Geometry check sheet. Reference: the model listing, model coordinates, mm. Face numbers are marked on the shaded views. A direction names the side the tool comes from. Coordinates: 2 decimals unless noted, no trailing zeros. Loops run counter-clockwise (first coordinate to the right, second up) from the corner with the lowest first, then second, coordinate; pieces in that order, holes last.
from build123d import *

# Parameters (mm, degrees)
F0_R        = 1.85
F0_R_2      = 15
F0_W        = 10
F0_H        = 10
F1_DEPTH    = 5
F2_DEPTH    = 22
F3_R        = 4.99999
F4_T1_DEPTH = 22
F5_R        = 1.5
F6_DEPTH    = 25


# Not quite as in the source:
# - a fillet or chamfer that OpenCascade refuses, or shapes differently, is made with other operations: its cross-section is extruded or revolved along the edge and cut away or added
# - a fillet or chamfer is up to 0.001 mm smaller than in the source, because OpenCascade refuses the exact size
# - a feature names something its author has since deleted; it is built from what else it names


with BuildPart() as f1:
    # F0 (on Top) → F1 (new body)
    with BuildSketch(Plane.XY):
        with BuildLine():
            Line((0, 15), (0, 0))
            Line((0, 0), (15, 0))
            Line((15, 0), (15, 3))
            ThreePointArc((15, 3), (8.6554793841, 7.8795661534), (5, 15))
            Line((5, 15), (0, 15))
        make_face()
        with Locations((6, 6)):
            Circle(F0_R, mode=Mode.SUBTRACT)
        with BuildLine():
            Line((15, 3), (15, 0))
            Line((15, 0), (35, 0))
            Line((35, 0), (35, 3))
            ThreePointArc((35, 3), (41.3445206159, 7.8795661534), (45, 15))
            Line((45, 15), (50, 15))
            Line((50, 15), (50, 35))
            Line((50, 35), (40, 35))
            Line((40, 35), (40, 45))
            Line((40, 45), (50, 45))
            Line((50, 45), (50, 100))
            Line((50, 100), (40, 100))
            Line((40, 100), (40, 104))
            Line((40, 104), (10, 104))
            Line((10, 104), (10, 100))
            Line((10, 100), (0, 100))
            Line((0, 100), (0, 45))
            Line((0, 45), (10, 45))
            Line((10, 45), (10, 35))
            Line((10, 35), (0, 35))
            Line((0, 35), (0, 15))
            Line((0, 15), (5, 15))
            ThreePointArc((5, 15), (8.6554793841, 7.8795661534), (15, 3))
        make_face()
        with Locations((25, 21.983)):
            Circle(F0_R_2, mode=Mode.SUBTRACT)
        with BuildLine():
            Line((15, 100), (35, 100))
            ThreePointArc((35, 100), (38.5355339059, 98.5355339059), (40, 95))
            Line((40, 95), (40, 55))
            ThreePointArc((40, 55), (38.5355339059, 51.4644660941), (35, 50))
            Line((35, 50), (15, 50))
            ThreePointArc((15, 50), (11.4644660941, 51.4644660941), (10, 55))
            Line((10, 55), (10, 95))
            ThreePointArc((10, 95), (11.4644660941, 98.5355339059), (15, 100))
        make_face(mode=Mode.SUBTRACT)
        with BuildLine():
            Line((35, 3), (35, 0))
            Line((35, 0), (50, 0))
            Line((50, 0), (50, 15))
            Line((50, 15), (45, 15))
            ThreePointArc((45, 15), (41.3445206159, 7.8795661534), (35, 3))
        make_face()
        with Locations((44, 6)):
            Circle(F0_R, mode=Mode.SUBTRACT)
        Polygon((0, 110), (0, 100), (10, 100), (10, 104), (40, 104), (40, 100), (50, 100), (50, 110), align=None)
        with Locations((6, 104)):
            Circle(F0_R, mode=Mode.SUBTRACT)
        with Locations((44, 104)):
            Circle(F0_R, mode=Mode.SUBTRACT)
        with Locations((5, 40)):
            Rectangle(F0_W, F0_H)
        with Locations((6, 40)):
            Circle(F0_R, mode=Mode.SUBTRACT)
        with Locations((45, 40)):
            Rectangle(F0_W, F0_H)
        with Locations((44, 40)):
            Circle(F0_R, mode=Mode.SUBTRACT)
    extrude(amount=F1_DEPTH)

    # F0 (on Top) → F2 (join)
    with BuildSketch(Plane.XY):
        with BuildLine():
            Line((35, 3), (35, 0))
            Line((35, 0), (50, 0))
            Line((50, 0), (50, 15))
            Line((50, 15), (45, 15))
            ThreePointArc((45, 15), (41.3445206159, 7.8795661534), (35, 3))
        make_face()
        with Locations((44, 6)):
            Circle(F0_R, mode=Mode.SUBTRACT)
        with BuildLine():
            Line((0, 15), (0, 0))
            Line((0, 0), (15, 0))
            Line((15, 0), (15, 3))
            ThreePointArc((15, 3), (8.6554793841, 7.8795661534), (5, 15))
            Line((5, 15), (0, 15))
        make_face()
        with Locations((6, 6)):
            Circle(F0_R, mode=Mode.SUBTRACT)
        with Locations((45, 40)):
            Rectangle(F0_W, F0_H)
        with Locations((44, 40)):
            Circle(F0_R, mode=Mode.SUBTRACT)
        with Locations((5, 40)):
            Rectangle(F0_W, F0_H)
        with Locations((6, 40)):
            Circle(F0_R, mode=Mode.SUBTRACT)
        Polygon((0, 110), (0, 100), (10, 100), (10, 104), (40, 104), (40, 100), (50, 100), (50, 110), align=None)
        with Locations((6, 104)):
            Circle(F0_R, mode=Mode.SUBTRACT)
        with Locations((44, 104)):
            Circle(F0_R, mode=Mode.SUBTRACT)
    extrude(amount=-F2_DEPTH)

    # F3 (radius 5 in the source; OpenCascade refuses exactly that, so slightly less here)
    f3_edges = [f1.edges().sort_by_distance(p)[0] for p in [
        (50, 0, -8.5),
        (0, 0, -8.5),
        (40, 35, -11),
        (40, 45, -11),
        (10, 35, -11),
        (10, 45, -11),
    ]]
    fillet(f3_edges, radius=F3_R)

    # F4: fillet of radius 5 on 2 edges, made by hand

    # F4_s2 → F4_t1 (join)
    with BuildSketch(Plane.XY.offset(-22)):
        with BuildLine():
            ThreePointArc((35.1010205144, 104), (38.2632981746, 102.8729833462), (40, 100))
            Line((40, 100), (40, 104))
            Line((40, 104), (35.1010205144, 104))
        make_face()
        with BuildLine():
            ThreePointArc((10, 100), (11.7367018254, 102.8729833462), (14.8989794856, 104))
            Line((14.8989794856, 104), (10, 104))
            Line((10, 104), (10, 100))
        make_face()
    extrude(amount=F4_T1_DEPTH)

    # F5 (on face) → F6 (cut)
    with BuildSketch(Plane(origin=(0, 110, 0), x_dir=(-1, 0, 0), z_dir=(0, 1, 0))):
        with Locations((-35, -15)):
            Circle(F5_R)
        with Locations((-35, -5)):
            Circle(F5_R)
        with Locations((-15, -5)):
            Circle(F5_R)
        with Locations((-15, -15)):
            Circle(F5_R)
        with Locations((-25, -15)):
            Circle(F5_R)
        with Locations((-25, -5)):
            Circle(F5_R)
    extrude(amount=-F6_DEPTH, mode=Mode.SUBTRACT)


solid = f1.part
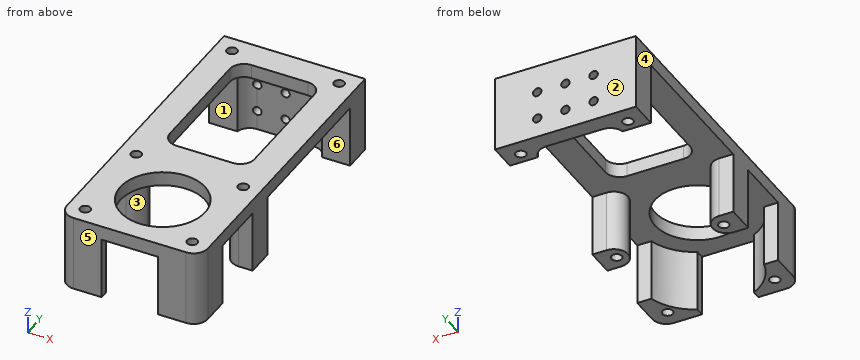
(1) Draft check along Y on the marked faces 4, 5 and 6. Enter one of: +Y half, -Y half, draft (parallel to the pull), parting line (faces both ways), or undercut.
Findings:
face 4: draft
face 5: -Y half
face 6: undercut
(2) Sectioned sample at C-C on z = -18.5. State how many separate pieces and enclosed holes the cut face has, and give its area (3 significant figures).
Findings:
separate pieces: 5
enclosed holes: 6
area: 786 mm2
(3) Gauge pin test, flat ends, axial feed: pin 1 Ø8 at (x, z) = (30.5, -17.5) entering from -Y; pin 2 Ø3 at (x, y) = (6, 6) entering from +Z (1 decimal); pin 3 Ø4 at (x, z) = (16.5, -10) entering from -Y; pin 4 Ø0.9 at (y, z) = (1.5, -12.5) entering from +X. Record the tip position at first contact, or that the pin passes through.
Findings:
pin 1: stops at y = 104
pin 2: passes through
pin 3: stops at y = 0
pin 4: stops at x = 48.96
(4) Sectioned sample at A-A on y = 88.5. Record the cut outline in (x, z).
Findings:
outline: (0, 0) - (10, 0) - (10, 5) - (0, 5) - close; (40, 0) - (50, 0) - (50, 5) - (40, 5) - close
(5) Sectioned sample at B-B on x = 25.5. Record the cut outline in (y, z), and give its area (3 significant figures).
Findings:
outline: (0, 0) - (6.99, 0) - (6.99, 5) - (0, 5) - close; (36.97, 0) - (50, 0) - (50, 5) - (36.97, 5) - close; (100, 0) - (104, 0) - (104, -3.59) - (110, -3.59) - (110, 5) - (100, 5) - close; (104, -22) - (110, -22) - (110, -16.41) - (104, -16.41) - close; (104, -13.59) - (110, -13.59) - (110, -6.41) - (104, -6.41) - close
area: 248 mm2
(6) Scan lines: L1, parallel to X at y = 104, z = 1.1; L2, parallel to Z at x = 25, y = 106.5; L3, parallel to Y at x = 3.5, z = -9. Record each from-to range of solid material in increasing order.
Findings:
L1: x = 0 to 4.15, 7.85 to 42.15, 45.85 to 50
L2: z = -22 to -16.5, -13.5 to -6.5, -3.5 to 5
L3: y = 0.23 to 15, 35 to 45, 100 to 110
(7) Access from +Z, -Z, +X, -X, +Y, -Y to the whole of each face (thin tool, end or side, straight path). Record for the marked faces 1, 2 and 3.
Findings:
face 1: -Z, +X, -X
face 2: +Z, -Z, +X, -X, +Y
face 3: -Z
